Read the model definition and answer for the solid it produces. Units are mm, in the model's axes. A direction names the side the tool comes from. Give positions to 0.01 mm unless a question says otherwise; leave off trailing zeros. Write each loop counter-clockwise with the first axis right and the second up, starting at its lowest first coordinate (ties: lowest second). Pieces come first, ordered by that corner, then holes. Notation, with made-up numbers: (48.25, -13) -> (63.25, -13) arc R21 ccw to (63.25, 22) -> close; hole circle Ø11 at (50.25, 32.5). An arc over 180 degrees is marked (long way). Use a Markdown table: item, result.
from build123d import *

# Parameters (mm, degrees)
SALIENTE_EXTRUIR1_DEPTH = 5
CORTAR_EXTRUIR1_DEPTH   = 5
CROQUIS3_W              = 76.666666666
CROQUIS3_H              = 5
CORTAR_EXTRUIR2_DEPTH   = 10
CROQUIS4_R              = 2.5
CORTAR_EXTRUIR3_DEPTH   = 10


with BuildPart() as part:
    # Croquis1 → Saliente-Extruir1 (new body)
    with BuildSketch(Plane.XY):
        Polygon((76.666666667, 5), (76.666666667, 0), (153.333333333, 0), (153.333333333, 5), (225, 5), (225, 21.666666667), (230, 21.666666667), (230, 38.333333333), (225, 38.333333333), (225, 55), (5, 55), (5, 38.333333333), (0, 38.333333333), (0, 21.666666667), (5, 21.666666667), (5, 5), align=None)
    extrude(amount=SALIENTE_EXTRUIR1_DEPTH)

    # Croquis2 → Cortar-Extruir1 (cut)
    with BuildSketch(Plane.XY.offset(5)):
        Polygon((35.833333333, 5), (35.833333333, 8.5), (34.333333333, 8.5), (34.333333333, 11.3), (35.833333333, 11.3), (35.833333333, 14), (40.833333333, 14), (40.833333333, 11.3), (42.333333333, 11.3), (42.333333333, 8.5), (40.833333333, 8.5), (40.833333333, 5), align=None)
        Polygon((189.166666667, 5), (189.166666667, 8.5), (187.666666667, 8.5), (187.666666667, 11.3), (189.166666667, 11.3), (189.166666667, 14), (194.166666667, 14), (194.166666667, 11.3), (195.666666667, 11.3), (195.666666667, 8.5), (194.166666667, 8.5), (194.166666667, 5), align=None)
    extrude(amount=-CORTAR_EXTRUIR1_DEPTH, mode=Mode.SUBTRACT)

    # Croquis3 → Cortar-Extruir2 (cut)
    with BuildSketch(Plane.XY.offset(5)):
        with Locations((115, 52.5)):
            Rectangle(CROQUIS3_W, CROQUIS3_H)
    extrude(amount=-CORTAR_EXTRUIR2_DEPTH, mode=Mode.SUBTRACT)

    # Croquis4 → Cortar-Extruir3 (cut)
    with BuildSketch(Plane.XY.offset(5)):
        with Locations((100, 25)):
            Circle(CROQUIS4_R)
        with Locations((130, 25)):
            Circle(CROQUIS4_R)
    extrude(amount=-CORTAR_EXTRUIR3_DEPTH, mode=Mode.SUBTRACT)


solid = part.part
Item 1: A cutting plane is placed at D-D (x = 38). Give the vertices of the cut face in (y, z), then the cut area to 3 significant figures.
Return value:
| item | result |
|---|---|
| outline | (14, 0) -> (55, 0) -> (55, 5) -> (14, 5) -> close |
| area | 205 mm^2 |
Item 2: A cutting plane is placed at C-C (z = 3.1). Count the separate pieces of the cut face and the enclosed holes in it, then the cut area to 3 significant figures.
Return value:
| item | result |
|---|---|
| separate pieces | 1 |
| enclosed holes | 2 |
| area | 11,000 mm^2 |
Item 3: A tool of negligible diameter and unlimited length cuts with its end or side. For faces 5 (the face through (228, 38.333, 2)), 6 (the face through (171, 5, 2)), 7 (the face through (5, 13, 2)), from which of +Z, -Z, +X, -X, +Y, -Y can it reach the whole face along a straight path? Write none if from no direction.
Return value:
| item | result |
|---|---|
| face 5 | +Z, -Z, +X, +Y |
| face 6 | +Z, -Z, +X, -Y |
| face 7 | +Z, -Z, -X, -Y |
Item 4: A cutting plane is placed at B-B (y = 25). Give the vertices of the cut face in (x, z), then the cut area to 3 significant figures.
Return value:
| item | result |
|---|---|
| outline | (0, 0) -> (97.5, 0) -> (97.5, 5) -> (0, 5) -> close; (102.5, 0) -> (127.5, 0) -> (127.5, 5) -> (102.5, 5) -> close; (132.5, 0) -> (230, 0) -> (230, 5) -> (132.5, 5) -> close |
| area | 1,100 mm^2 |
Item 5: Each of these flat-tipped pins is pushed along its axis until it touches: P1, Ø2, axis at y = 10, z = 3.5, coming from the -X side; P2, Ø2.5, axis at y = 53.5, z = 3, coming from the +X side; P3, Ø2.5, axis at x = 227, z = 3.5, coming from the +Y side. Where does it stop, or does it pass through?
Return value:
| item | result |
|---|---|
| P1 | x = 5 |
| P2 | x = 225 |
| P3 | y = 38.33 |
Item 6: A cutting plane is placed at A-A (x = 130). Give the vertices of the cut face in (y, z).
Return value:
| item | result |
|---|---|
| outline | (0, 0) -> (22.5, 0) -> (22.5, 5) -> (0, 5) -> close; (27.5, 0) -> (50, 0) -> (50, 5) -> (27.5, 5) -> close |
Item 7: For a pull along X with two mould halves and no side action, classify faces 1 (the face through (153.333, 52, 3)), 2 (the face through (76.667, 52, 3)), 3 (the face through (5, 47, 2)), 4 (the face through (230, 30, 2)) as +X half, -X half, draft (parallel to the pull), parting line (faces both ways), or undercut.
Return value:
| item | result |
|---|---|
| face 1 | undercut |
| face 2 | undercut |
| face 3 | -X half |
| face 4 | +X half |
Item 8: Straight lines are drawn through the part: line 1 along X through (y, z) = (5.5, 4.3); line 2 along X through (y, z) = (11, 2); line 3 along Y through (x, z) = (130, 3.25). For each, find the intervals that lie inside material, in ascending order. Write a range as [from, to].
Return value:
| item | result |
|---|---|
| line 1 | [5, 35.83], [40.83, 189.17], [194.17, 225] |
| line 2 | [5, 34.33], [42.33, 187.67], [195.67, 225] |
| line 3 | [0, 22.5], [27.5, 50] |
